Part model, mm, in its own coordinate system. A direction names the side the tool comes from. Coordinates: 2 decimals unless noted, no trailing zeros. Write each loop counter-clockwise with the first axis right and the second up, starting at its lowest first coordinate (ties: lowest second). Pieces come first, ordered by that corner, then holes. Notation, with made-up numbers: (84.5, 15.5) - (107.5, 15.5) arc R21 ccw to (107.5, 45.5) - close; hole circle Ø1 at (87.25, -34). An arc over 180 degrees is marked (long way). Use a Markdown table: item, result.
```python
from build123d import *

# Parameters (mm, degrees)
F0_W     = 150
F0_H     = 150
F0_W_2   = 67.5
F0_H_2   = 67.5
F1_DEPTH = 150
F3_DEPTH = 42
F5_DEPTH = 50


with BuildPart() as f1:
    # F0 (on Front) → F1 (new body)
    with BuildSketch(Plane.XZ):
        with Locations((75, 75)):
            Rectangle(F0_W, F0_H)
        with Locations((38.75, 38.75)):
            Rectangle(F0_W_2, F0_H_2, mode=Mode.SUBTRACT)
        with Locations((111.25, 38.75)):
            Rectangle(F0_W_2, F0_H_2, mode=Mode.SUBTRACT)
        with Locations((38.75, 111.25)):
            Rectangle(F0_W_2, F0_H_2, mode=Mode.SUBTRACT)
        with Locations((111.25, 111.25)):
            Rectangle(F0_W_2, F0_H_2, mode=Mode.SUBTRACT)
    extrude(amount=F1_DEPTH)

    # F2 (on face) → F3 (join)
    with BuildSketch(Plane.YZ.offset(150)):
        Polygon((0, 150), (-75, 150), (-150, 66.9503435493), (-75.0411003828, 84.2106193304), (-41.5993146598, 41.4914414287), (-69.6472600102, 15.3852747753), (-55.3271184714, 0), (0, 0), align=None)
    extrude(amount=F3_DEPTH)

    # F4 (on face) → F5 (join)
    with BuildSketch(Plane.XY.offset(150)):
        Polygon((78.8858830929, -47.45561257), (52.7330078185, 0), (0, 0), (0, -150), (150, -150), (150, -75), (192, -75), (192, -60.3085644543), (151.335395945, -14.7103952784), (154.8433154821, -44.6645244956), (108.5957586765, -112.5511825085), (7.5965225697, -138.2962316275), (4.1573755443, -63.4704530239), (11.035669595, -122.2042143345), (11.035669595, -24.9770767987), (34.6234440804, -112.5511825085), (34.6234440804, -53.7799745798), (94.1806063056, -87.2614681721), (136.4469230175, -27.8326813132), align=None)
    extrude(amount=F5_DEPTH)


solid = f1.part
```
Item 1: Which spindle directions (+Z, -Z, +X, -X, +Y, -Y) get a long thin tool onto all of the face, cutting with end or side? Do faces 1 (the face through (171, -75, 175)), 2 (the face through (65.993, -24.06, 174.65)), 3 (the face through (111, -74, 5)). Say none if no direction does.
From the geometry:
| item | result |
|---|---|
| face 1 | +Z, +X, -Y |
| face 2 | +Z, +Y |
| face 3 | +Y, -Y |
Item 2: Drill centre lines: probe 1 along X at (y, z) = (-132.5, 119); probe 2 along Z at (x, y) = (60.5, -15). Where is each one in solid material? Low to high.
From the geometry:
| item | result |
|---|---|
| probe 1 | 0 to 5, 72.5 to 77.5, 145 to 150 |
| probe 2 | 0 to 5, 72.5 to 77.5, 145 to 200 |
Item 3: Band-saw the part on C-C, the plane y = -119. Count the separate pieces of the cut face and the enclosed holes in it, then the cut area to 3 significant figures.
From the geometry:
| item | result |
|---|---|
| separate pieces | 1 |
| enclosed holes | 4 |
| area | 9,110 mm^2 |
Item 4: Band-saw the part on D-D, the plane z = 55.5. Give the cut face in (x, y), then the cut area to 3 significant figures.
From the geometry:
| item | result |
|---|---|
| outline | (0, -150) - (5, -150) - (5, 0) - (0, 0) - close; (72.5, -150) - (77.5, -150) - (77.5, 0) - (72.5, 0) - close; (145, -150) - (150, -150) - (150, -52.57) - (192, -52.57) - (192, 0) - (145, 0) - close |
| area | 4,460 mm^2 |
Item 5: Two-plate mould, pull along Z, no slides. Class faces 4 (the face through (73, -74, 200)), 5 (the face through (38, -74, 72.5)), 6 (the face through (108.069, -37.507, 174.65)): pulls with the +Z half, pulls with the -Z half, needs draft (parallel to the pull), parting line crosses it, or undercut.
From the geometry:
| item | result |
|---|---|
| face 4 | pulls with the +Z half |
| face 5 | undercut |
| face 6 | needs draft |
Item 6: Band-saw the part on A-A, the plane x = 133.5. Give the cut face in (y, z).
From the geometry:
| item | result |
|---|---|
| outline | (-150, 0) - (0, 0) - (0, 5) - (-150, 5) - close; (-150, 72.5) - (0, 72.5) - (0, 77.5) - (-150, 77.5) - close; (-150, 145) - (0, 145) - (0, 150) - (-28.84, 150) - (-28.84, 200) - (-31.98, 200) - (-31.98, 150) - (-75.99, 150) - (-75.99, 200) - (-150, 200) - close |
Item 7: Drop a flat-ended pin along its axis: P1, Ø1, axis at y = -130.5, z = 23.5, coming from the +X side. Give the stop position or say it passes through.
From the geometry:
| item | result |
|---|---|
| P1 | x = 150 |
Item 8: Band-saw the part on B-B, the plane z = 184. Give the cut face in (x, y), then the cut area to 3 significant figures.
From the geometry:
| item | result |
|---|---|
| outline | (0, -150) - (150, -150) - (150, -75) - (192, -75) - (192, -60.31) - (151.34, -14.71) - (154.84, -44.66) - (108.6, -112.55) - (7.6, -138.3) - (4.16, -63.47) - (11.04, -122.2) - (11.04, -24.98) - (34.62, -112.55) - (34.62, -53.78) - (94.18, -87.26) - (136.45, -27.83) - (78.89, -47.46) - (52.73, 0) - (0, 0) - close |
| area | 13,700 mm^2 |
